```python
from build123d import *

# Parameters (mm, degrees)
SKETCH1_W           = 102
SKETCH1_H           = 32
BOSS_EXTRUDE1_DEPTH = 1
SKETCH2_W           = 102
SKETCH2_H           = 32
SKETCH2_W_2         = 101
SKETCH2_H_2         = 31
BOSS_EXTRUDE2_DEPTH = 3
SKETCH3_R           = 1.75
CUT_EXTRUDE1_DEPTH  = 107.943910533
FILLET1_R           = 3
SKETCH4_R           = 6
CUT_EXTRUDE2_DEPTH  = 107.976632963


with BuildPart() as part:
    # Sketch1 → Boss-Extrude1 (new body)
    with BuildSketch(Plane.XY):
        with Locations((-51, 16)):
            Rectangle(SKETCH1_W, SKETCH1_H)
    extrude(amount=BOSS_EXTRUDE1_DEPTH)

    # Sketch2 → Boss-Extrude2 (add)
    # profile 1 of 2: a face of its own
    with BuildSketch(Plane.XY.offset(1)):
        with Locations((-51, 16)):
            Rectangle(SKETCH2_W, SKETCH2_H)
        with Locations((-51, 16)):
            Rectangle(SKETCH2_W_2, SKETCH2_H_2, mode=Mode.SUBTRACT)
    # profile 2 of 2: a face of its own
    with BuildSketch(Plane.XY.offset(1)):
        with BuildLine():
            Line((-97.5, 14.527864045), (-97.5, 4.5))
            Line((-97.5, 4.5), (-4.5, 4.5))
            Line((-4.5, 4.5), (-4.5, 14.527864045))
            ThreePointArc((-4.5, 14.527864045), (-9.5, 19), (-4.5, 23.472135955))
            Line((-4.5, 23.472135955), (-4.5, 27.5))
            Line((-4.5, 27.5), (-97.5, 27.5))
            Line((-97.5, 27.5), (-97.5, 23.472135955))
            ThreePointArc((-97.5, 23.472135955), (-92.5, 19), (-97.5, 14.527864045))
        make_face()
    extrude(amount=BOSS_EXTRUDE2_DEPTH)

    # Sketch3 → Cut-Extrude1 (cut, through all)
    with BuildSketch(Plane.XY.offset(1)):
        with Locations((-97, 19)):
            Circle(SKETCH3_R)
        with Locations((-5, 19)):
            Circle(SKETCH3_R)
    extrude(amount=-CUT_EXTRUDE1_DEPTH, mode=Mode.SUBTRACT)

    # Fillet1
    fillet1_edges = [part.edges().sort_by_distance(p)[0] for p in [
        (-101.5, 31.5, 2.5),
        (-0.5, 31.5, 2.5),
        (-0.5, 0.5, 2.5),
        (-101.5, 0.5, 2.5),
        (0, 0, 2),
        (-102, 0, 2),
        (-102, 32, 2),
        (0, 32, 2),
    ]]
    fillet(fillet1_edges, radius=FILLET1_R)

    # Sketch4 → Cut-Extrude2 (cut, through all)
    with BuildSketch(Plane(origin=(0, 0, 0), x_dir=(-1, 0, 0), z_dir=(0, 0, -1))):
        with Locations((26, 18.94)):
            Circle(SKETCH4_R)
        with Locations((76, 18.94)):
            Circle(SKETCH4_R)
    extrude(amount=-CUT_EXTRUDE2_DEPTH, mode=Mode.SUBTRACT)


solid = part.part
```
Geometry check sheet. Reference: the model listing, model coordinates, mm. A direction names the side the tool comes from. Give positions to 0.01 mm unless a question says otherwise; leave off trailing zeros. Order: outer loops, then holes, each group sorted by start corner. A loop starts at its lowest first (then second) coordinate and runs counter-clockwise, first axis right, second up. Notation, with made-up numbers: (69.25, -22.5) - (111.25, -22.5) arc R26 cw to (111.25, 15.5) - close; hole circle Ø11 at (6.5, 57). An arc over 180 degrees is marked (long way). Answer in a Markdown table with one row per item. Add a question column.
Q1. Cross-section at C-C, the plane x = -42. Enter the section's corners in (y, z), then the cut area to 3 significant figures.
Q2. Gauge pin test, flat end, axial feed: pin 1 (11.5 mm diameter, centred on x = -5, y = 19, fed in from +Z). Record the tip position at first contact, or that the pin passes through.
Q3. Cross-section at B-B, the plane y = 8. Enter the section's corners in (x, z), then the cut area to 3 significant figures.
Q4. Mould release check, pull along Y, two halves, no side actions. Record for faces 3 (the flat face through (-97.5, 26, 2)), 4 (the flat face through (-52, 32, 2)), 5 (the cylindrical face through (-0.9, 0.86, 2.03)): pulls with the +Y half, pulls with the -Y half, needs draft (parallel to the pull), parting line crosses it, or undercut.
Q5. Material ranges on probe 1 along X at (y, z) = (25, 3.2); probe 2 along X at (y, z) = (19, 2.6); probe 3 along Y at (x, z) = (-97, 0.25), recorded low to high. Write a range as from..to.
Q6. Tool access check on faces 1 (the flat face through (-97.5, 10, 2)), 2 (the flat face through (-52, 0, 2)). Record the directions out of +Z, -Z, +X, -X, +Y, -Y that give a thin tool (end or side, any length) a straight path to the whole face; none if there is none.
Q7. Cross-section at A-A, the plane x = -26. Enter the section's corners in (y, z).
Check values:
| question | item | result |
|---|---|---|
| 1 | outline | (0, 0) - (32, 0) - (32, 4) - (31.5, 4) - (31.5, 1) - (27.5, 1) - (27.5, 4) - (4.5, 4) - (4.5, 1) - (0.5, 1) - (0.5, 4) - (0, 4) - close |
| 1 | area | 104 mm^2 |
| 2 | pin 1 | stops at z = 4 |
| 3 | outline | (-102, 0) - (0, 0) - (0, 4) - (-0.5, 4) - (-0.5, 1) - (-4.5, 1) - (-4.5, 4) - (-97.5, 4) - (-97.5, 1) - (-101.5, 1) - (-101.5, 4) - (-102, 4) - close |
| 3 | area | 384 mm^2 |
| 4 | face 3 | undercut |
| 4 | face 4 | pulls with the +Y half |
| 4 | face 5 | pulls with the -Y half |
| 5 | probe 1 | x = -102..-101.5, -97.5..-4.5, -0.5..0 |
| 5 | probe 2 | x = -102..-101.5, -92.5..-82, -70..-32, -20..-9.5, -0.5..0 |
| 5 | probe 3 | y = 0..17.25, 20.75..32 |
| 6 | face 1 | +Z |
| 6 | face 2 | +Z, -Z, +X, -X, -Y |
| 7 | outline | (0, 0) - (12.94, 0) - (12.94, 4) - (4.5, 4) - (4.5, 1) - (0.5, 1) - (0.5, 4) - (0, 4) - close; (24.94, 0) - (32, 0) - (32, 4) - (31.5, 4) - (31.5, 1) - (27.5, 1) - (27.5, 4) - (24.94, 4) - close |
